The figure shows three views and two pictorial views of one solid part (mm, origin at its lowest corner). Answer the questions. Coordinates: 2 decimals unless noted, no trailing zeros. Write each loop counter-clockwise with the first axis right and the second up, starting at its lowest first coordinate (ties: lowest second). Pieces come first, ordered by that corner, then holes. Notation, with made-up numbers: M 53,65.5 L 65,65.5 A24 cw 65,80.5 Z; hole C -3.5,55.25 d5. An arc over 180 degrees is marked long. Write item = value, one per line.
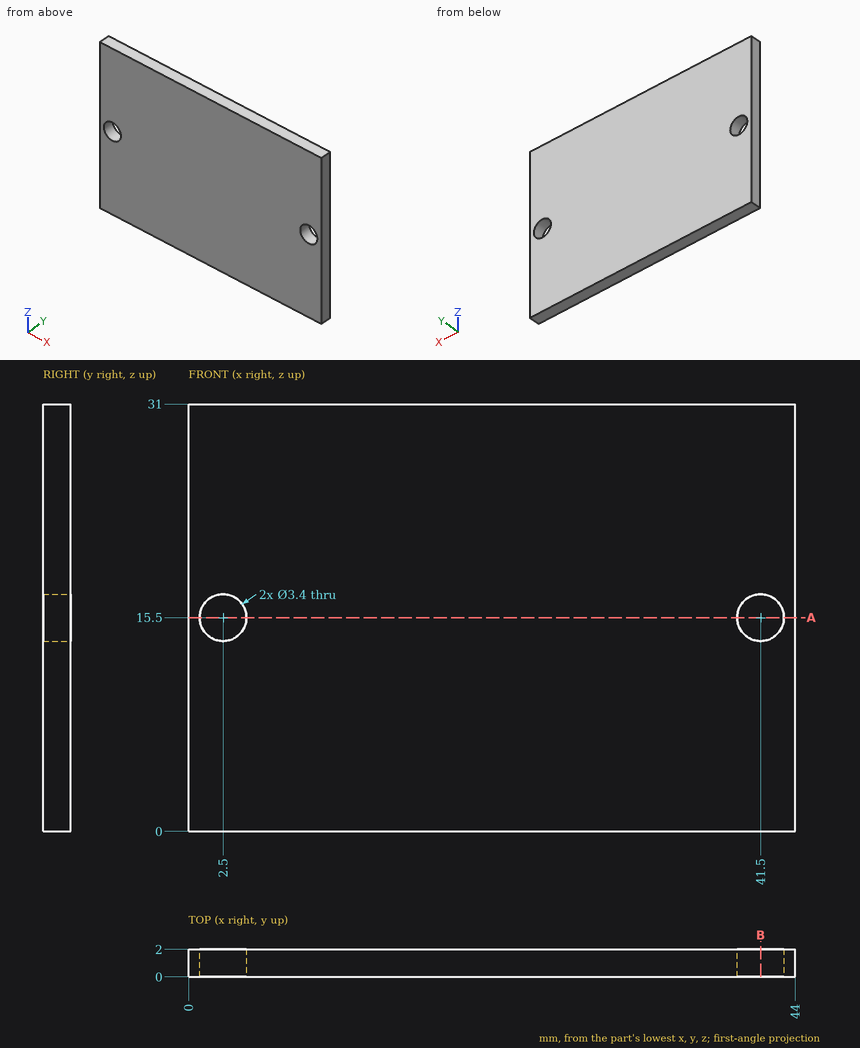
Item 1: Consider line 1 along X through (y, z) = (1.25, 15.5); line 2 along Z through (x, y) = (41.5, 0.8); line 3 along X through (y, z) = (0.2, 14). Determine where each line is inside the solid, lowest interval first. Write a range as from..to.
Worked answers:
line_1 = 0..0.8, 4.2..39.8, 43.2..44
line_2 = 0..13.8, 17.2..31
line_3 = 0..1.7, 3.3..40.7, 42.3..44
Item 2: Find section B-B (x = 41.5). Determine the outline of the cut face in (y, z), and give its area (3 significant figures).
Worked answers:
outline = M 0,0 L 2,0 L 2,13.8 L 0,13.8 Z; M 0,17.2 L 2,17.2 L 2,31 L 0,31 Z
area = 55.2 mm²
Item 3: Find section A-A (z = 15.5). Determine the outline of the cut face in (x, y).
Worked answers:
outline = M 0,0 L 0.8,0 L 0.8,2 L 0,2 Z; M 4.2,0 L 39.8,0 L 39.8,2 L 4.2,2 Z; M 43.2,0 L 44,0 L 44,2 L 43.2,2 Z
